Here's how the part is built. I have some questions about the finished solid (model axes, mm). A direction names the side the tool comes from. Give positions to 0.01 mm unless a question says otherwise; leave off trailing zeros. Loops run counter-clockwise (first coordinate to the right, second up) from the corner with the lowest first, then second, coordinate; pieces in that order, holes last. Notation, with made-up numbers: M 5,36 L 16,36 A36 cw 16,74 Z; hole C -9.5,21 d6. An arc over 180 degrees is marked long. Answer as CSV lines item,"result". Start each with the question number.
Item 1: Will these pins go through, and if not, where does the flat tip stop? P1, Ø8, axis at x = -76, z = 3.5, coming from the -Y side; P2, Ø1.8, axis at x = 5, y = 3.5, coming from the +Z side; P3, Ø4, axis at y = 4, z = 5.5, coming from the +X side.
Item 2: I want a section at B-B on x = -56. List the corners of the cut face in (y, z) for me.
Item 3: If I drill on line 1 along X through (y, z) = (7, 2.5); line 2 along X through (y, z) = (72, 6); line 3 along X through (y, z) = (76.5, 2.5), over which ranges is the centre line in solid material (lowest first)? Write a range as from..to.
Item 4: I want a section at A-A on y = 44. List the corners of the cut face in (x, z) for me, plus the area to 3 significant figures.
Item 5: If we mould it in two halves opening along Z, with no side actions, what happens to faces 5 (the flat face through (-125, 90, 0)), 6 (the cylindrical face through (0, -0.2, -7.5)), 7 (the cylindrical face through (-58.41, 9.54, 3))? For each: released by +Z, released by -Z, zero draft, split by the parting line, or undercut.
Item 6: For faces 1 (the cylindrical face through (-135, 58, 0)), 2 (the flat face through (-9, 12, 0)), 3 (the cylindrical face through (72.97, 9.54, 3)), 4 (the cylindrical face through (7.5, -0.2, 0)), which set-ups out of +Z, -Z, +X, -X, +Y, -Y let a thin tool reach every point of the face, with its end or its side?
from build123d import *

# Parameters (mm, degrees)
SKETCH_2_R               = 9.999999999999993
FILLET_1_R               = 5
CUT_EXTRUDE_1_DEPTH      = 165.01524327634917
CUT_EXTRUDE_1_DEPTH_BACK = 165.01524327634917


with BuildPart() as part:
    # По траектории1: sweep along a path in Эскиз1
    with BuildLine(Plane.XY) as sweep_1_path:
        Line((-125, 90), (-125, 31.999999999999993))
        ThreePointArc((-125, 31.999999999999993), (-115.62741699796952, 9.372583002030478), (-93, 0))
        Line((-93, 0), (124.99999999999999, 0))
    # Эскиз2 → По траектории1 (sweep)
    with BuildSketch(Plane(origin=(0, 90, 0), x_dir=(1, 0, 0), z_dir=(0, 1, 0))):
        with Locations((-125, 0)):
            Circle(SKETCH_2_R)
    sweep(path=sweep_1_path.line)

    # Эскиз3 → Повернуть1 (revolve)
    with BuildSketch(Plane.XY):
        with BuildLine():
            Line((4.49e-15, 12), (4.49e-15, -12))
            Line((4.49e-15, -12), (-20.784609690826528, -12))
            ThreePointArc((-20.784609690826528, -12), (-24, 2.94e-15), (-20.784609690826528, 12))
            Line((-20.784609690826528, 12), (4.49e-15, 12))
        make_face()
    revolve(axis=Axis((4.49e-15, 20.353481922740002, 0), (-1.1e-16, -1, 0)))

    # Эскиз6 → Вырез-Повернуть1 (revolve, cut)
    with BuildSketch(Plane.XY, mode=Mode.PRIVATE) as cut_revolve_1_sk:
        with BuildLine():
            Line((123.3345611656252, 10.000000000000009), (253.93494063523158, 10.000000000000009))
            Line((253.93494063523158, 10.000000000000009), (253.93494063523158, 0))
            Line((253.93494063523158, 0), (124.58650256653851, 0))
            ThreePointArc((124.58650256653851, 0), (124.89155809301906, 5.116559027883884), (123.3345611656252, 10.000000000000009))
        make_face()
    revolve(cut_revolve_1_sk.sketch.rotate(Axis((-23.23871769146635, 0, 0), (1, 0, 0)), 90), axis=Axis((-23.23871769146635, 0, 0), (1, 0, 0)), mode=Mode.SUBTRACT)

    # Скругление1
    fillet_1_edges = [part.edges().sort_by_distance(p)[0] for p in [
        (-135, 90, 1.22e-15),
    ]]
    fillet(fillet_1_edges, radius=FILLET_1_R)
    fillet_1_2_edges = [part.edges().sort_by_distance(p)[0] for p in [
        (-21.81742422927143, 2.45e-15, 9.999999999999993),
        (-21.81742422927143, -1.22e-15, -9.999999999999993),
    ]]
    fillet(fillet_1_2_edges, radius=FILLET_1_R - 0.0001)  # a hair under: the kernel refuses the full size
    fillet_1_3_edges = [part.edges().sort_by_distance(p)[0] for p in [
        (21.817424229271403, -9.999999999999993, 3.06e-15),
    ]]
    fillet(fillet_1_3_edges, radius=FILLET_1_R)
    fillet_1_4_edges = [part.edges().sort_by_distance(p)[0] for p in [
        (123.33456116562522, 7.071067811865514, 7.071067811865446),
        (123.33456116562522, -7.07106781186551, -7.071067811865451),
    ]]
    fillet(fillet_1_4_edges, radius=FILLET_1_R)

    # Эскиз7 → Вырез-Вытянуть1 (cut, two sides: drawn at the far end of the back side and taken through both)
    with BuildSketch(Plane(origin=(0, 0, 0), x_dir=(1, 0, 0), z_dir=(0, 1, 0)).offset(-CUT_EXTRUDE_1_DEPTH_BACK)):
        with BuildLine():
            ThreePointArc((-6.999999999999877, -6.273754856543386), (-6.646803743153483, -6.646803743153611), (-6.273754856543252, -6.999999999999998))
            Line((-6.273754856543248, -7.000000000000002), (-2.6925824035672585, -7.000000000000006))
            ThreePointArc((-2.692582403567258, -6.999999999999998), (-3.242e-14, -7.5), (2.6925824035671977, -7.000000000000021))
            Line((2.692582403567193, -7.000000000000002), (6.2737548565430865, -7.000000000000002))
            ThreePointArc((6.273754856543118, -7.000000000000118), (6.646803743153469, -6.646803743153625), (6.999999999999976, -6.273754856543277))
            Line((6.999999999999987, -6.273754856543277), (6.999999999999956, -2.6925824035677124))
            ThreePointArc((6.999999999999835, -2.692582403567684), (7.500000000000001, 1.33e-15), (6.999999999999835, 2.6925824035676857))
            Line((6.999999999999997, 2.692582403567716), (6.999999999999997, 6.27375485654329))
            ThreePointArc((6.999999999999971, 6.273754856543282), (6.646803743153472, 6.6468037431536215), (6.273754856543124, 7.000000000000112))
            Line((6.2737548565430865, 6.999999999999998), (2.6925824035671964, 6.999999999999998))
            ThreePointArc((2.6925824035671995, 7.000000000000021), (-3.331e-14, 7.500000000000001), (-2.692582403567263, 6.9999999999999964))
            Line((-2.692582403567263, 7.0000000000000036), (-6.27375485654325, 6.999999999999999))
            ThreePointArc((-6.273754856543249, 7), (-6.646803743153482, 6.646803743153612), (-6.999999999999876, 6.273754856543388))
            Line((-7.000000000000003, 6.273754856543425), (-7.000000000000003, 2.692582403567693))
            ThreePointArc((-6.999999999999842, 2.692582403567664), (-7.5, -2.22e-15), (-6.99999999999984, -2.692582403567666))
            Line((-6.99999999999992, -2.6925824035676946), (-6.999999999999922, -6.273754856543425))
        make_face()
    extrude(amount=CUT_EXTRUDE_1_DEPTH + CUT_EXTRUDE_1_DEPTH_BACK, mode=Mode.SUBTRACT)


solid = part.part
Result:
1,P1,"y = -10"
1,P2,"z = 23.43"
1,P3,"x = 124.93"
2,outline,"C 0,0 d20"
3,line 1,"-126.35..-7.07, 7.07..124.22"
3,line 2,"-133..-117"
3,line 3,"-134.68..-115.32"
4,outline,"C -125,0 d20"
4,area,"314 mm^2"
5,face 5,"zero draft"
5,face 6,"undercut"
5,face 7,"split by the parting line"
6,face 1,"+Y"
6,face 2,"+Z, -Z, +X, +Y"
6,face 3,"+X"
6,face 4,"+Y, -Y"
